from build123d import *

# Parameters (mm, degrees)
BOSS_EXTRUDE1_DEPTH      = 30
BOSS_EXTRUDE2_DEPTH      = 5
BOSS_EXTRUDE2_DEPTH_BACK = 5
FILLET1_R                = 10
FILLET2_R                = 1


with BuildPart() as part:
    # Sketch2 → Boss-Extrude1 (new body)
    with BuildSketch(Plane.XY):
        Polygon((0, 0), (-5, 0), (-5, 10), (10, 10), (10, -45), (-5, -45), (-5, -35), (0, -35), (0, -37.5), (-2.5, -37.5), (-2.5, -42.5), (7.5, -42.5), (7.5, 7.5), (-2.5, 7.5), (-2.5, 2.5), (0, 2.5), align=None)
    extrude(amount=BOSS_EXTRUDE1_DEPTH)

    # Sketch3 → Boss-Extrude2 (add, two sides: drawn at the far end of the back side and taken through both)
    with BuildSketch(Plane(origin=(0, -17.5, 0), x_dir=(-1, 0, 0), z_dir=(0, -1, 0)).offset(-BOSS_EXTRUDE2_DEPTH_BACK)):
        Polygon((-10, -6), (-60, -30), (-10, -30), align=None)
    extrude(amount=BOSS_EXTRUDE2_DEPTH + BOSS_EXTRUDE2_DEPTH_BACK)

    # Fillet1
    # the kernel refuses this fillet: 10 mm, written as the material it adds along each edge
    with BuildSketch(Plane(origin=(10, -22.5, 6), x_dir=(0, 0, -1), z_dir=(0, 1, 0))) as fillet1_piece_1:
        with BuildLine():
            CenterArc((6.294420553, -9.995664887), FILLET1_R, 91.687149317, 62.671844859)
            Line((-2.720810021, -5.668354211), (0, 0))
            Line((0, 0), (6, 0))
        make_face()
    extrude(amount=10)
    with BuildSketch(Plane(origin=(10, -12.5, 30), x_dir=(0, 1, 0), z_dir=(0, 0, -1))) as fillet1_piece_2_section:
        with BuildLine():
            CenterArc((FILLET1_R, FILLET1_R), FILLET1_R, 180, 90)
            Line((0, FILLET1_R), (0, 0))
            Line((0, 0), (FILLET1_R, 0))
        make_face()
    fillet1_piece_2 = extrude(amount=49, mode=Mode.PRIVATE)
    fillet1_piece_2 = split(fillet1_piece_2, bisect_by=Plane(origin=(19.362808843, -12.5, 10.494148244), z_dir=(-0.4327310675847713, 0, 0.9015230574682737)), keep=Keep.TOP, mode=Mode.PRIVATE)
    add(fillet1_piece_2)
    with BuildSketch(Plane(origin=(10, -22.5, 30), x_dir=(0, -1, 0), z_dir=(0, 0, -1))) as fillet1_piece_3_section:
        with BuildLine():
            CenterArc((FILLET1_R, -FILLET1_R), FILLET1_R, 90, 90)
            Line((0, -FILLET1_R), (0, 0))
            Line((0, 0), (FILLET1_R, 0))
        make_face()
    fillet1_piece_3 = extrude(amount=49, mode=Mode.PRIVATE)
    fillet1_piece_3 = split(fillet1_piece_3, bisect_by=Plane(origin=(19.362808843, -22.5, 10.494148244), z_dir=(-0.4327310675847713, 0, 0.9015230574682737)), keep=Keep.TOP, mode=Mode.PRIVATE)
    add(fillet1_piece_3)
    with BuildSketch(Plane(origin=(10, -22.5, 30), x_dir=(0, -1, 0), z_dir=(0, 0, -1))) as fillet1_piece_4a_section:
        with BuildLine():
            CenterArc((FILLET1_R, -FILLET1_R), FILLET1_R, 90, 90)
            Line((0, -FILLET1_R), (0, 0))
            Line((0, 0), (FILLET1_R, 0))
        make_face()
    fillet1_piece_4a = extrude(amount=49, mode=Mode.PRIVATE)
    fillet1_piece_4a = split(fillet1_piece_4a, bisect_by=Plane(origin=(10, -22.5, 0), z_dir=(0, 0, 1)), keep=Keep.TOP, mode=Mode.PRIVATE)
    fillet1_piece_4a = split(fillet1_piece_4a, bisect_by=Plane(origin=(19.362808843, -22.5, 10.494148244), z_dir=(0.4327310675847713, 0, -0.9015230574682737)), keep=Keep.TOP, mode=Mode.PRIVATE)
    with BuildSketch(Plane(origin=(10, -38.218827612, 6), x_dir=(0, 0, -1), z_dir=(0, 1, 0))) as fillet1_piece_4b_section:
        with BuildLine():
            CenterArc((6.294420553, -9.995664887), FILLET1_R, 91.687149317, 62.671844859)
            Line((-2.720810021, -5.668354211), (0, 0))
            Line((0, 0), (6, 0))
        make_face()
    fillet1_piece_4b = extrude(amount=25.718827612, mode=Mode.PRIVATE)
    fillet1_piece_4b = split(fillet1_piece_4b, bisect_by=Plane(origin=(10, -22.5, 6), z_dir=(0, -1, 0)), keep=Keep.TOP, mode=Mode.PRIVATE)
    fillet1_piece_4 = fillet1_piece_4a & fillet1_piece_4b
    add(fillet1_piece_4)
    with BuildSketch(Plane(origin=(10, -22.5, 6), x_dir=(0, 0, -1), z_dir=(0, 1, 0))) as fillet1_piece_5a_section:
        with BuildLine():
            CenterArc((6.294420553, -9.995664887), FILLET1_R, 91.687149317, 62.671844859)
            Line((-2.720810021, -5.668354211), (0, 0))
            Line((0, 0), (6, 0))
        make_face()
    fillet1_piece_5a = extrude(amount=25.718827612, mode=Mode.PRIVATE)
    fillet1_piece_5a = split(fillet1_piece_5a, bisect_by=Plane(origin=(10, -12.5, 6), z_dir=(0, 1, 0)), keep=Keep.TOP, mode=Mode.PRIVATE)
    with BuildSketch(Plane(origin=(10, -12.5, 30), x_dir=(0, 1, 0), z_dir=(0, 0, -1))) as fillet1_piece_5b_section:
        with BuildLine():
            CenterArc((FILLET1_R, FILLET1_R), FILLET1_R, 180, 90)
            Line((0, FILLET1_R), (0, 0))
            Line((0, 0), (FILLET1_R, 0))
        make_face()
    fillet1_piece_5b = extrude(amount=49, mode=Mode.PRIVATE)
    fillet1_piece_5b = split(fillet1_piece_5b, bisect_by=Plane(origin=(10, -12.5, 0), z_dir=(0, 0, 1)), keep=Keep.TOP, mode=Mode.PRIVATE)
    fillet1_piece_5b = split(fillet1_piece_5b, bisect_by=Plane(origin=(19.362808843, -12.5, 10.494148244), z_dir=(0.4327310675847713, 0, -0.9015230574682737)), keep=Keep.TOP, mode=Mode.PRIVATE)
    fillet1_piece_5 = fillet1_piece_5a & fillet1_piece_5b
    add(fillet1_piece_5)

    # Fillet2
    fillet2_edges = [part.edges().sort_by_distance(p)[0] for p in [
        (60, -17.5, 30),
    ]]
    fillet(fillet2_edges, radius=FILLET2_R)


solid = part.part
Geometry: final body of the model. Coordinates: model frame, mm. A direction names the side the tool comes from. Give positions to 0.01 mm unless a question says otherwise; leave off trailing zeros. Loops run counter-clockwise (first coordinate to the right, second up) from the corner with the lowest first, then second, coordinate; pieces in that order, holes last. Notation, with made-up numbers: M 51.25,78.5 L 93.25,78.5 A19 cw 93.25,110.5 Z; hole C 11,55 d1. An arc over 180 degrees is marked long. Put each result on its own line as item: value. Start each with the question number.
1) Cut plane D-D (x = 27.5). Output: boundary loops of the cut face in (y, z).
2) Cut plane B-B (z = 27). Output: boundary loops of the cut face in (x, y).
3) Access query for faces 4 (the flat face through (-1, -37.5, 15)), 5 (the flat face through (-3, -35, 15)), 6 (the flat face through (10, 4, 15)). Directions: +Z, -Z, +X, -X, +Y, -Y. A direction counts if a zero-diameter tool reaches every point of the face in a straight line with its end or side. Return the directions, or none.
4) Cut plane C-C (y = -20.5). Output: boundary loops of the cut face in (x, z).
5) Pull-direction query (Y, two-part tool) for faces 1 (the flat face through (2, 10, 15)), 2 (the flat face through (-2.5, 5, 15)), 3 (the flat face through (-5, 5, 15)); classes: pulls with the +Y half, pulls with the -Y half, needs draft (parallel to the pull), parting line crosses it, or undercut.
6) Cut plane A-A (x = 5.5). Output: boundary loops of the cut face in (y, z).
7) Ray query, line 1 along Y through (x, z) = (-0.5, 28); line 2 along X through (y, z) = (3, 24.5); line 3 along Y through (x, z) = (5, 5). Return the intervals inside material, ascending.
8) Contact query for flat-ended pins moving along their axis: pin 1 (9 mm diameter, centred on y = -18, z = 14, fed in from -X); pin 2 (6 mm diameter, centred on x = 41, z = 25, fed in from +Y); pin 3 (14 mm diameter, centred on y = -41.5, z = 9.5, fed in from +X). Output: stop coordinate, or through.
Verdict:
1. outline: M -22.5,14.4 L -12.5,14.4 L -12.5,30 L -22.5,30 Z
2. outline: M -5,-45 L 10,-45 L 10,-32.5 A10 cw 20,-22.5 L 53.75,-22.5 L 53.75,-12.5 L 20,-12.5 A10 cw 10,-2.5 L 10,10 L -5,10 L -5,0 L 0,0 L 0,2.5 L -2.5,2.5 L -2.5,7.5 L 7.5,7.5 L 7.5,-42.5 L -2.5,-42.5 L -2.5,-37.5 L 0,-37.5 L 0,-35 L -5,-35 Z
3. face 4: +Z, -Z
3. face 5: +Z, -Z, -X
3. face 6: +Z, -Z, +X, +Y
4. outline: M 7.5,0 L 10,0 A10 cw 15.67,8.72 L 56.04,28.1 A1 ccw 55.61,30 L 7.5,30 Z
5. face 1: pulls with the +Y half
5. face 2: undercut
5. face 3: needs draft
6. outline: M -45,0 L -42.5,0 L -42.5,30 L -45,30 Z; M 7.5,0 L 10,0 L 10,30 L 7.5,30 Z
7. line 1: -45 to -42.5, -37.5 to -35, 0 to 2.5, 7.5 to 10
7. line 2: -5 to -2.5, 7.5 to 10
7. line 3: -45 to -42.5, 7.5 to 10
8. pin 1: x = 7.5
8. pin 2: y = -12.5
8. pin 3: x = 10
